Work out the finished part from the listing and answer in its coordinate system (mm). Give positions to 0.01 mm unless a question says otherwise; leave off trailing zeros. Loops run counter-clockwise (first coordinate to the right, second up) from the corner with the lowest first, then second, coordinate; pieces in that order, holes last. Notation, with made-up numbers: (9.25, -15) - (18.25, -15) arc R22 ccw to (18.25, 21) - close; hole circle Ø2 at (-25.75, 27). An arc over 180 degrees is marked (long way). One line per item, written item: value.
Autodesk Inventor part; units mm, degrees
ref_plane "YZ Plane" through (0, 0, 0) normal (1, 0, 0) x (0, 1, 0)
ref_plane "XZ Plane" through (0, 0, 0) normal (0, 1, 0) x (-1, 0, 0)
ref_plane "XY Plane" through (0, 0, 0) normal (0, 0, 1) x (1, 0, 0)
sketch "Эскиз1" plane through (0, 0, 0) normal (1, 0, 0) x (0, 1, 0)
  line L0 (0, 0) -> (10.522, 0) construction
  line L1 (0, 0) -> (0, -19) construction
  line L2 (0, 0) -> (0, -27.3) construction
  line L3 (0, -19) -> (3, -19)
  line L4 (3, -19) -> (3, -27.3)
  line L5 (3, -27.3) -> (0, -27.3)
  line L6 (0, -27.3) -> (0, -19)
  dimension "d0" = 19
  dimension "d1" = 27.3
  dimension "d2" = 3
revolve "Вращение1" add sketch "Эскиз1" angle 360 about axis through (0, 0, 0) along (0, 1, 0)
chamfer "Фаска1" distance 2 angle 45 1 edges at (0, 3, 19) measured on face at (2.1778, 3, -24.2689)
chamfer "Фаска2" distance 2 angle 45 1 edges at (0, 3, 27.3) measured on face at (3.853, 3, -24.7322)
sketch "Эскиз2" plane through (0, 0, 0) normal (1, 0, 0) x (0, 1, 0)
  line L0 (0, 0) -> (7.8289, 0) construction
  line L1 (0, 0) -> (0, -24.8) construction
  line L2 (0, 27.3) -> (0, -27.3) construction
  line L3 (0, -25.3) -> (-2.8173, -25.3)
  line L4 (0, -27.3) -> (-2.5558, -27.3)
  line L5 (-3.0173, -25.3) -> (-3.0173, -26.7) construction
  line L6 (0, -25.3) -> (0, -27.3)
  line L7 (-4.0346, 0.25) -> (-4.0346, -25) construction
  line L8 (-4.0346, -25) -> (-6, -25) construction
  arc A0 (-3.2173, -25.1) -> (-4.4555, -26.5989) centre (-4.0173, -25.7) ccw
  line L9 (-5.0173, -25) -> (-5.0173, 0) construction
  line L10 (-4.0346, -24.7) -> (-5.0173, -24.7) construction
  line L11 (-3.0173, -25.3) -> (-3.1008, -25.3) construction
  arc A1 (-3.0173, -25.7) -> (-3.1008, -25.3) centre (-4.0173, -25.7) ccw construction
  arc A2 (-3.2173, -25.1) -> (-2.8173, -25.3) centre (-2.8173, -24.8) ccw
  line L12 (-3.4322, -27.0978) -> (-4.4555, -26.5989)
  arc A3 (-4.4555, -26.5989) -> (-3.0173, -25.7) centre (-4.0173, -25.7) ccw construction
  arc A4 (-3.4322, -27.0978) -> (-2.5558, -27.3) centre (-2.5558, -25.3) ccw
  point P0 (-3.3032, -25)
  point P1 (-3.0173, -27.3)
  dimension "d10" = 24.8
  dimension "d11" = 3.017
  dimension "d12" = 0.5
  dimension "d14" = 4.035
  dimension "d15" = 2
  dimension "d16" = 0.983
  dimension "d17" = 0.3
  dimension "d18" = 0.5
  dimension "d19" = 50
  dimension "d21" = 3.017
  dimension "d22" = 2
revolve "Вращение2" add sketch "Эскиз2" angle 45 about axis through (0, 0, 0) along (0, -1, 0)
pattern_circular "Круговой массив1" count 4 over 360 about axis through (0, 1.5, 0) along (0, -1, 0) of "Вращение2"
properties part number "mirror_lock_v3"
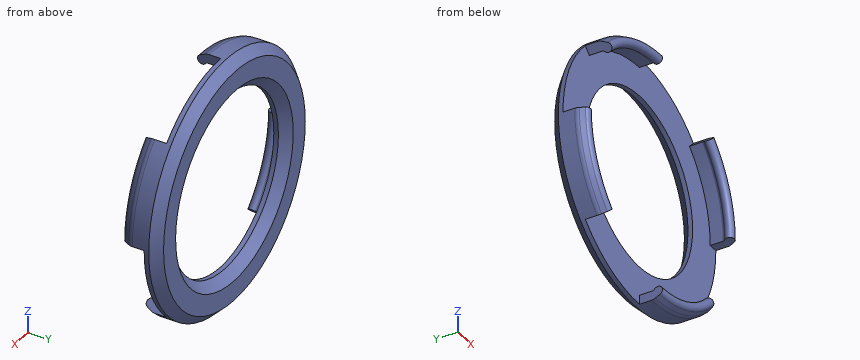
1. Flat-ended cylindrical pins translate along their axes: pin 1 Ø1.5 at (y, z) = (-2.5, -6.5) entering from -X; pin 2 Ø1.3 at (x, y) = (26.5, -3.5) entering from -Z; pin 3 Ø1.5 at (x, y) = (0.5, -3.5) entering from +Z. Find the tip coordinate at first contact, or state that the pin passes through.
Output:
pin 1: stops at x = -26.69
pin 2: stops at z = 0
pin 3: stops at z = 27.26
2. Find the intervals of material crossed by line 1 along Z through (x, y) = (0, 0.65); line 2 along X through (y, z) = (-0.75, 18), in increasing order.
Output:
line 1: z = -27.3 to -19, 19 to 27.3
line 2: x = -18 to -17.78, 18 to 20.53
3. Section A-A (y = 2) is taken. Write down the section's boundary in (x, z).
Output:
outline: circle Ø52.6 at (0, 0); hole circle Ø40 at (0, 0)
